The listing builds one solid part. Answer for the finished solid, in the listing's coordinates (mm). A direction names the side the tool comes from. Round coordinates to 2 decimals unless told otherwise and drop trailing zeros. Write each loop counter-clockwise with the first axis right and the second up, starting at its lowest first coordinate (ties: lowest second). Pieces come first, ordered by that corner, then holes. Notation, with made-up numbers: (4.25, 10.5) - (25.25, 10.5) arc R18 cw to (25.25, 22.5) - close; hole circle Ø8 at (-38.75, -33.5). An arc over 180 degrees is marked (long way). Answer in a Markdown table with one row per item.
from build123d import *

# Parameters (mm, degrees)
F0_W     = 139.7
F0_H     = 177.8
F1_DEPTH = 9.525
F0_W_2   = 63.5
F0_R     = 1.905
F2_DEPTH = 17.78
F3_SIZE  = 2.54
F4_SIZE  = 0.508
F5_R     = 5.08
F6_W     = 19.05
F6_H     = 15.875
F7_DEPTH = 5.08


with BuildPart() as f1:
    # F0 (on Top) → F1 (new body)
    with BuildSketch(Plane.XY):
        with Locations((-31.75, 0)):
            Rectangle(F0_W, F0_H)
    extrude(amount=F1_DEPTH)

    # F0 (on Top) → F2 (join)
    with BuildSketch(Plane.XY):
        with Locations((69.85, 0)):
            Rectangle(F0_W_2, F0_H)
        with Locations((53.975, -63.5)):
            Circle(F0_R, mode=Mode.SUBTRACT)
        with Locations((85.725, -63.5)):
            Circle(F0_R, mode=Mode.SUBTRACT)
        with Locations((53.975, 0)):
            Circle(F0_R, mode=Mode.SUBTRACT)
        with Locations((85.725, 0)):
            Circle(F0_R, mode=Mode.SUBTRACT)
        with Locations((53.975, 63.5)):
            Circle(F0_R, mode=Mode.SUBTRACT)
        with Locations((85.725, 63.5)):
            Circle(F0_R, mode=Mode.SUBTRACT)
    extrude(amount=F2_DEPTH)

    # F3
    f3_edges = [f1.edges().sort_by_distance(p)[0] for p in [
        (52.07, -63.5, 0),
        (83.82, -63.5, 0),
        (52.07, 0, 0),
        (83.82, 0, 0),
        (52.07, 63.5, 0),
        (83.82, 63.5, 0),
    ]]
    chamfer(f3_edges, length=F3_SIZE)

    # F4
    f4_edges = [f1.edges().sort_by_distance(p)[0] for p in [
        (0, -88.9, 0),
        (101.6, 0, 0),
        (0, 88.9, 0),
        (-101.6, 0, 0),
    ]]
    chamfer(f4_edges, length=F4_SIZE)

    # F5
    f5_edges = [f1.edges().sort_by_distance(p)[0] for p in [
        (-31.75, -88.9, 9.525),
        (-101.6, 0, 9.525),
        (-31.75, 88.9, 9.525),
    ]]
    fillet(f5_edges, radius=F5_R)

    # F6 (on face) → F7 (cut)
    with BuildSketch(Plane.XY.offset(17.78)):
        with Locations((47.625, -38.1)):
            Rectangle(F6_W, F6_H)
    extrude(amount=-F7_DEPTH, mode=Mode.SUBTRACT)


solid = f1.part
(1) Find the intervals of material crossed by line 1 (Y direction, x = -12, z = 5); line 2 (Y direction, x = 54.5, z = 12.5); line 3 (Z direction, x = -59.5, y = 67.5) (3 decimals), in increasing order.
Checked values:
| item | result |
|---|---|
| line 1 | y = -88.87 to 88.87 |
| line 2 | y = -88.9 to -65.33, -61.67 to -1.83, 1.83 to 61.67, 65.33 to 88.9 |
| line 3 | z = 0 to 9.525 |
(2) Flat-ended cylindrical pins translate along their axes: pin 1 (1 mm diameter, centred on y = -25.5, z = 12.5, fed in from -X); pin 2 (5 mm diameter, centred on x = 21.5, y = -68.5, fed in from +Z) (3 decimals); pin 3 (1.5 mm diameter, centred on y = -15.5, z = 9, fed in from -X). Find the tip coordinate at first contact, or state that the pin passes through.
Checked values:
| item | result |
|---|---|
| pin 1 | stops at x = 38.1 |
| pin 2 | stops at z = 9.525 |
| pin 3 | stops at x = -99.89 |
(3) For faces 4 (the cylindrical face through (-30.77, 87.45, 8)), 5 (the conical face through (85.3, -65.5, 2.4)), 6 (the flat face through (-30, 1, 9.525)), 7 (the flat face through (47, -46.038, 15)), determine the directions among +Z, -Z, +X, -X, +Y, -Y from which every point of the face is accessible in a straight line to the end or side of a thin tool.
Checked values:
| item | result |
|---|---|
| face 4 | +Z, -X, +Y |
| face 5 | -Z |
| face 6 | +Z, -X, +Y, -Y |
| face 7 | +Z, -X |
(4) For a pull along Y with two mould halves and no side action, classify faces 1 (the cylindrical face through (-30.77, -87.45, 8)), 2 (the cylindrical face through (-100.15, 1.24, 8)), 3 (the flat face through (47, -38, 12.7)) as pulls with the +Y half, pulls with the -Y half, needs draft (parallel to the pull), parting line crosses it, or undercut.
Checked values:
| item | result |
|---|---|
| face 1 | pulls with the -Y half |
| face 2 | needs draft |
| face 3 | undercut |
(5) Section A-A (x = -33) is taken. Give the vertices of the cut face in (y, z) (3 decimals), and give its area (3 significant figures).
Checked values:
| item | result |
|---|---|
| outline | (-88.9, 0.508) - (-88.392, 0) - (88.392, 0) - (88.9, 0.508) - (88.9, 4.445) arc R5.08 ccw to (83.82, 9.525) - (-83.82, 9.525) arc R5.08 ccw to (-88.9, 4.445) - close |
| area | 1,680 mm2 |
(6) Section B-B (y = 19.5) is taken. Give the vertices of the cut face in (x, z) (3 decimals), and give its area (3 significant figures).
Checked values:
| item | result |
|---|---|
| outline | (-101.6, 0.508) - (-101.092, 0) - (101.092, 0) - (101.6, 0.508) - (101.6, 17.78) - (38.1, 17.78) - (38.1, 9.525) - (-96.52, 9.525) arc R5.08 ccw to (-101.6, 4.445) - close |
| area | 2,450 mm2 |
